The listing builds one solid part. Answer for the finished solid, in the listing's coordinates (mm). Face numbers are marked on the shaded views. A direction names the side the tool comes from. Give positions to 0.01 mm unless a question says otherwise; leave off trailing zeros. Order: outer loops, then holes, each group sorted by start corner. A loop starts at its lowest first (then second) coordinate and runs counter-clockwise, first axis right, second up.
```python
from build123d import *

# Parameters (mm, degrees)
SKETCH_1_W          = 56
SKETCH_1_H          = 16
EXTRUDE_1_DEPTH     = 3
SKETCH_3_R          = 1.6
CUT_EXTRUDE_2_DEPTH = 5
FILLET_1_R          = 2
EXTRUDE_2_DEPTH     = 3
SKETCH_5_R          = 0.6
SKETCH_5_W          = 9
SKETCH_5_H          = 16
EXTRUDE_3_DEPTH     = 3
EXTRUDE_5_DEPTH     = 1.5
EXTRUDE_6_DEPTH     = 1.5
EXTRUDE_7_DEPTH     = 9


with BuildPart() as part:
    # 草图1 → 凸台-拉伸1 (new body)
    with BuildSketch(Plane(origin=(0, 0, 0), x_dir=(1, 0, 0), z_dir=(0, 1, 0))):
        Rectangle(SKETCH_1_W, SKETCH_1_H)
    extrude(amount=EXTRUDE_1_DEPTH)

    # 草图3 → 切除-拉伸2 (cut)
    with BuildSketch(Plane(origin=(0, 3, 0), x_dir=(1, 0, 0), z_dir=(0, 1, 0))):
        with Locations(Location((23.5, 0, 0), (0, 0, 270))):
            Circle(SKETCH_3_R)
        with Locations(Location((-23.5, 0, 0), (0, 0, 270))):
            Circle(SKETCH_3_R)
    extrude(amount=-CUT_EXTRUDE_2_DEPTH, mode=Mode.SUBTRACT)

    # 圆角1
    fillet_1_edges = [part.edges().sort_by_distance(p)[0] for p in [
        (28, 1.5, 8),
        (-28, 1.5, 8),
        (-28, 1.5, -8),
        (28, 1.5, -8),
    ]]
    fillet(fillet_1_edges, radius=FILLET_1_R)

    # 草图4 → 凸台-拉伸2 (add)
    with BuildSketch(Plane(origin=(0, 3, 0), x_dir=(1, 0, 0), z_dir=(0, 1, 0))):
        with BuildLine():
            Line((0, -8), (0, -18))
            Line((0, -18), (5, -18))
            ThreePointArc((5, -18), (5.707106781, -17.707106781), (6, -17))
            Line((6, -17), (6, -8))
            Line((6, -8), (0, -8))
        make_face()
        with BuildLine():
            Line((-5, -18), (0, -18))
            Line((0, -18), (0, -8))
            Line((0, -8), (-6, -8))
            Line((-6, -8), (-6, -17))
            ThreePointArc((-6, -17), (-5.707106781, -17.707106781), (-5, -18))
        make_face()
    extrude(amount=-EXTRUDE_2_DEPTH)

    # 草图5 → 凸台-拉伸3 (add)
    with BuildSketch(Plane.XY):
        with BuildLine():
            Line((-6, 3), (-6, 29))
            ThreePointArc((-6, 29), (-5.707106781, 29.707106781), (-5, 30))
            Line((-5, 30), (5, 30))
            ThreePointArc((5, 30), (5.707106781, 29.707106781), (6, 29))
            Line((6, 29), (6, 3))
            Line((6, 3), (-6, 3))
        make_face()
        with Locations((0, 7)):
            Circle(SKETCH_5_R, mode=Mode.SUBTRACT)
        with Locations(Location((0, 25, 0), (0, 0, 180))):
            Circle(SKETCH_5_R, mode=Mode.SUBTRACT)
        with Locations((0, 16)):
            Rectangle(SKETCH_5_W, SKETCH_5_H, mode=Mode.SUBTRACT)
    extrude(amount=EXTRUDE_3_DEPTH)

    # 草图7 → 凸台-拉伸5 (add)
    with BuildSketch(Plane(origin=(6, 0, 0), x_dir=(0, 0, -1), z_dir=(1, 0, 0))):
        Polygon((-3, 27), (-9.430780618, 3), (-3, 3), align=None)
    extrude(amount=-EXTRUDE_5_DEPTH)

    # 草图8 → 凸台-拉伸6 (add)
    with BuildSketch(Plane.ZY.offset(6)):
        Polygon((3, 27), (9.430780618, 3), (3, 3), align=None)
    extrude(amount=-EXTRUDE_6_DEPTH)

    # 草图9 → 凸台-拉伸7 (add)
    with BuildSketch(Plane.ZY.offset(-4.5)):
        with BuildLine():
            Line((3, 6), (3, 3))
            Line((3, 3), (6, 3))
            ThreePointArc((6, 3), (3.878679656, 3.878679656), (3, 6))
        make_face()
    extrude(amount=EXTRUDE_7_DEPTH)


solid = part.part
```
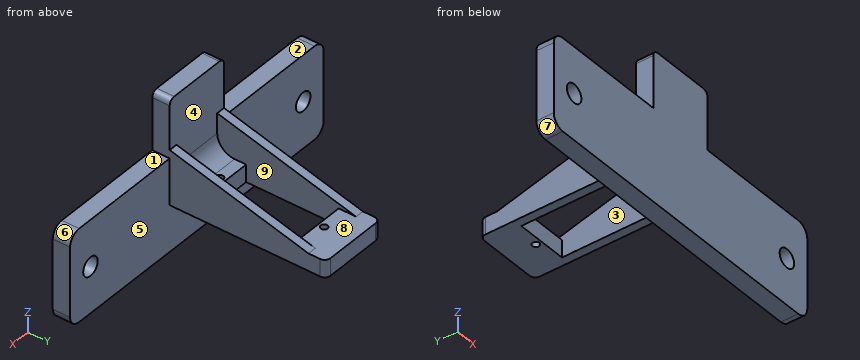
1) Find section C-C (z = -3.5). Write down the section's boundary in (x, y).
Geometry says:
outline: (-28, 0) - (28, 0) - (28, 3) - (-28, 3) - close
2) Straight lines are drawn through the part: probe 1 along Y at (x, z) = (0, 2.3); probe 2 along X at (y, z) = (2.3, 0); probe 3 along X at (y, z) = (25, 2.05). For each, find the intervals that lie inside material, in ascending order.
Geometry says:
probe 1: y = 0 to 6.4, 7.6 to 8, 24 to 24.4, 25.6 to 30
probe 2: x = -28 to -25.1, -21.9 to 21.9, 25.1 to 28
probe 3: x = -6 to -0.6, 0.6 to 6
3) Find section B-B (y = 12). Write down the section's boundary in (x, z), then the cut area to 3 significant figures.
Geometry says:
outline: (-6, 0) - (-4.5, 0) - (-4.5, 7.02) - (-6, 7.02) - close; (4.5, 0) - (6, 0) - (6, 7.02) - (4.5, 7.02) - close
area: 21.1 mm2
4) Find section A-A (x = 0). Write down the section's boundary in (y, z).
Geometry says:
outline: (0, -8) - (3, -8) - (3, 0) - (6.4, 0) - (6.4, 3) - (6, 3) arc R3 cw to (3, 6) - (3, 18) - (0, 18) - close; (7.6, 0) - (8, 0) - (8, 3) - (7.6, 3) - close; (24, 0) - (24.4, 0) - (24.4, 3) - (24, 3) - close; (25.6, 0) - (30, 0) - (30, 3) - (25.6, 3) - close
5) Given P1, Ø5, axis at y = 14.5, z = 0, coming from the +X side; P2, Ø8, axis at x = 17.5, z = 1, coming from the +Y side; P3, Ø2.5, axis at x = -23.5, z = 0, coming from the +Y side; P4, Ø6, axis at x = 0, y = 22.5, coming from the -Z side, each flat-ended and moving along its own axis, determine where each tip first touches the part or whether it passes through.
Geometry says:
P1: stops at x = 6
P2: stops at y = 3
P3: passes through
P4: stops at z = 0
6) A tool of negligible diameter and unlimited length cuts with its end or side. For the marked faces 1, 2, 3, 4 and 5, from which of +Z, -Z, +X, -X, +Y, -Y can it reach the whole face along a straight path? Write none if from no direction.
Geometry says:
face 1: +Z, +X, +Y, -Y
face 2: +Z, -X, +Y, -Y
face 3: +Z
face 4: +Z, +Y
face 5: -Z, +Y
7) Find section D-D (y = 17). Write down the section's boundary in (x, z).
Geometry says:
outline: (-6, 0) - (-4.5, 0) - (-4.5, 5.68) - (-6, 5.68) - close; (4.5, 0) - (6, 0) - (6, 5.68) - (4.5, 5.68) - close
8) For a pull along X with two mould halves and no side action, classify the marked faces 6, 7, 8 and 9 as +X half, -X half, draft (parallel to the pull), parting line (faces both ways), or undercut.
Geometry says:
face 6: +X half
face 7: -X half
face 8: undercut
face 9: undercut
